from build123d import *

# Parameters (mm, degrees)
F0_W     = 60
F0_H     = 60
F1_DEPTH = 5
F2_R     = 5
F4_DEPTH = 3
F3_R     = 5
F5_DEPTH = 4
F3_R_2   = 3
F6_DEPTH = 5
F3_W     = 20
F3_H     = 7.223957
F7_DEPTH = 2


with BuildPart() as f1:
    # F0 (on Top) → F1 (new body)
    with BuildSketch(Plane.XY):
        with Locations((30, -30)):
            Rectangle(F0_W, F0_H)
    extrude(amount=F1_DEPTH)

    # F2
    f2_edges = [f1.edges().sort_by_distance(p)[0] for p in [
        (60, 0, 2.5),
        (60, -60, 2.5),
    ]]
    fillet(f2_edges, radius=F2_R)

    # F3 (on face) → F4 (cut)
    with BuildSketch(Plane.XY.offset(5)):
        Polygon((40, -5), (5, -5), (5, -55), (40, -55), (40, -43.888409), (40, -36.664452), align=None)
    extrude(amount=-F4_DEPTH, mode=Mode.SUBTRACT)

    # F3 (on face) → F5 (cut)
    with BuildSketch(Plane.XY.offset(5)):
        with Locations((50, -10)):
            Circle(F3_R)
    extrude(amount=-F5_DEPTH, mode=Mode.SUBTRACT)

    # F3 (on face) → F6 (cut)
    with BuildSketch(Plane.XY.offset(5)):
        with Locations((50, -30)):
            Circle(F3_R_2)
    extrude(amount=-F6_DEPTH, mode=Mode.SUBTRACT)

    # F3 (on face) → F7 (cut)
    with BuildSketch(Plane.XY.offset(5)):
        with Locations((50, -40.27643)):
            Rectangle(F3_W, F3_H)
    extrude(amount=-F7_DEPTH, mode=Mode.SUBTRACT)


solid = f1.part
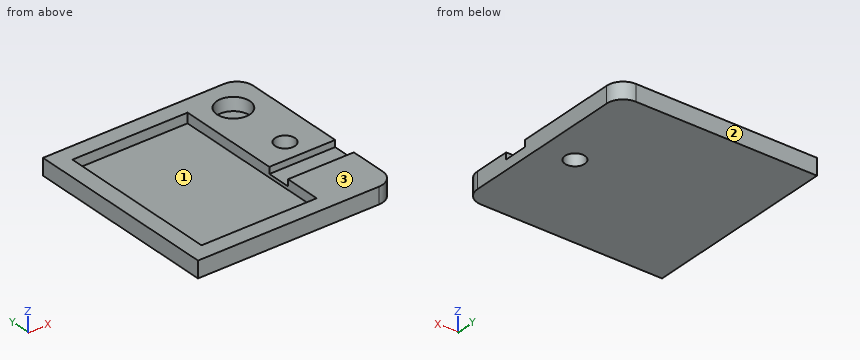
For this review, take the finished solid that the model builds, in its own axes (mm). Face numbers are marked on the shaded views. Round coordinates to 2 decimals unless told otherwise and drop trailing zeros. Loops run counter-clockwise (first coordinate to the right, second up) from the corner with the lowest first, then second, coordinate; pieces in that order, holes last. Notation, with made-up numbers: (7, -35) - (36, -35) arc R16 ccw to (36, -28) - close; hole circle Ø8 at (-37.5, 37.5). An arc over 180 degrees is marked (long way). Use one line per item in the form item = value.
1) We need section B-B on x = 50. Write out the cut boundary in (y, z), then the cut area to 3 significant figures.
Solutions:
outline = (-60, 0) - (-33, 0) - (-33, 5) - (-36.66, 5) - (-36.66, 3) - (-43.89, 3) - (-43.89, 5) - (-60, 5) - close; (-27, 0) - (0, 0) - (0, 5) - (-5, 5) - (-5, 1) - (-15, 1) - (-15, 5) - (-27, 5) - close
area = 216 mm2
2) We need section C-C on y = -51.5. Write out the cut boundary in (x, z).
Solutions:
outline = (0, 0) - (60, 0) - (60, 5) - (40, 5) - (40, 2) - (5, 2) - (5, 5) - (0, 5) - close
3) We need section D-D on x = 56.5. Write out the cut boundary in (y, z).
Solutions:
outline = (-59.77, 0) - (-0.23, 0) - (-0.23, 5) - (-36.66, 5) - (-36.66, 3) - (-43.89, 3) - (-43.89, 5) - (-59.77, 5) - close
4) Mouldability with a two-part tool opening along Y and no side actions: class the marked faces 1, 2 and 3 as pulls with the +Y half, pulls with the -Y half, needs draft (parallel to the pull), parting line crosses it, or undercut.
Solutions:
face_1 = undercut
face_2 = pulls with the +Y half
face_3 = needs draft
5) Wall thickness on probe 1 along Y at (x, z) = (50, 4.15); probe 2 along X at (y, z) = (-18.5, 3.75); probe 3 along X at (y, z) = (-31, 2.45): over which ranges is each line inside the solid? List them lowest first.
Solutions:
probe_1 = -60 to -43.89, -36.66 to -33, -27 to -15, -5 to 0
probe_2 = 0 to 5, 40 to 60
probe_3 = 0 to 5, 40 to 47.17, 52.83 to 60
6) We need section A-A on y = -30. Write out the cut boundary in (x, z), then the cut area to 3 significant figures.
Solutions:
outline = (0, 0) - (47, 0) - (47, 5) - (40, 5) - (40, 2) - (5, 2) - (5, 5) - (0, 5) - close; (53, 0) - (60, 0) - (60, 5) - (53, 5) - close
area = 165 mm2
7) Clearance check with flat-ended pins moving along their axes: P1, Ø5, axis at x = 50.5, y = -10.5, coming from the +Z side; P2, Ø4, axis at x = 32.5, y = -29, coming from the +Z side. State where each tip first meets the part, or that it passes through.
Solutions:
P1 = 1
P2 = 2
